```python
from build123d import *

# Parameters (mm, degrees)
F0_W      = 304.8
F0_H      = 41.91
F1_DEPTH  = 72.39
F3_DEPTH  = 44.45
F4_R      = 9.525
F5_DEPTH  = 52.07
F7_DEPTH  = 42.164
F9_DEPTH  = 43.18
F10_R     = 5.08
F11_R     = 5.08
F12_R     = 1.8364316327
F13_DEPTH = 50.8
F14_R     = 2.0092193571
F15_DEPTH = 50.8


with BuildPart() as f1:
    # F0 (on Top) → F1 (new body)
    with BuildSketch(Plane.XY):
        with Locations((152.4, 20.955)):
            Rectangle(F0_W, F0_H)
    extrude(amount=F1_DEPTH)

    # F2 (on face) → F3 (cut)
    with BuildSketch(Plane.XZ):
        Polygon((304.8, 72.39), (0, 72.39), (304.8, 19.05), align=None)
    extrude(amount=-F3_DEPTH, mode=Mode.SUBTRACT)

    # F4 (on face) → F5 (cut)
    with BuildSketch(Plane(origin=(0, 0, 0), x_dir=(0, -1, 0), z_dir=(-1, 0, 0))):
        with Locations((-20.955, 31.115)):
            Circle(F4_R)
    extrude(amount=-F5_DEPTH, mode=Mode.SUBTRACT)

    # F6 (on face) → F7 (cut)
    with BuildSketch(Plane.XZ):
        Polygon((0, 72.39), (0, 53.7492334843), (68.9350515604, 53.7492334843), (95.2856466174, 29.7941416502), (207.8745663166, 29.7941416502), (304.8, 0), (304.8, 19.05), align=None)
    extrude(amount=-F7_DEPTH, mode=Mode.SUBTRACT)

    # F8 (on face) → F9 (cut)
    with BuildSketch(Plane.XZ):
        Polygon((0, 53.7492334843), (0, 46.6843768954), (65.1628002524, 46.6843768954), (95.2856466174, 21.5315297246), (207.8745663166, 21.5315297246), (304.8, 0), (207.8745663166, 29.7941416502), (95.2856466174, 29.7941416502), (68.9350515604, 53.7492334843), align=None)
    extrude(amount=-F9_DEPTH, mode=Mode.SUBTRACT)

    # F10
    f10_edges = [f1.edges().sort_by_distance(p)[0] for p in [
        (152.4, 0, 0),
        (256.337283, 0, 10.765765),
        (151.580106, 0, 21.53153),
        (80.224223, 0, 34.107953),
        (32.5814, 0, 46.684377),
        (0, 0, 23.342188),
    ]]
    fillet(f10_edges, radius=F10_R)

    # F11
    f11_edges = [f1.edges().sort_by_distance(p)[0] for p in [
        (152.4, 41.91, 0),
        (0, 41.91, 23.342188),
        (32.5814, 41.91, 46.684377),
        (80.224223, 41.91, 34.107953),
        (151.580106, 41.91, 21.53153),
        (256.337283, 41.91, 10.765765),
    ]]
    fillet(f11_edges, radius=F11_R)

    # F12 (on face) → F13 (cut)
    with BuildSketch(Plane.XZ):
        with Locations((63.3207473448, 9.5940940082)):
            Circle(F12_R)
    extrude(amount=-F13_DEPTH, mode=Mode.SUBTRACT)

    # F14 (on face) → F15 (cut)
    with BuildSketch(Plane.XZ):
        with Locations((207.3171118243, 8.7452335283)):
            Circle(F14_R)
    extrude(amount=-F15_DEPTH, mode=Mode.SUBTRACT)


solid = f1.part
```
CAD build for the part. Positions are in the model's coordinates, mm. A direction names the side the tool comes from. Round coordinates to 2 decimals unless told otherwise and drop trailing zeros. Order: outer loops, then holes, each group sorted by start corner. A loop starts at its lowest first (then second) coordinate and runs counter-clockwise, first axis right, second up.
Item 1: Saw through at D-D on y = 8. Write the cut outline in (x, z).
Item 2: Saw through at B-B on y = 19.5. Write the cut outline in (x, z).
Item 3: Pin check, flat tips, straight feed: pin 1 (5 mm diameter, centred on x = 207.32, z = 8.75, fed in from +Y); pin 2 (16 mm diameter, centred on x = 154.5, y = 22, fed in from +Z); pin 3 (6 mm diameter, centred on y = 19.5, z = 33, fed in from -X). Stop position of each tip, or through.
Item 4: Saw through at A-A on x = 26.5. Write the cut outline in (y, z) (3 decimals), then the cut area to 3 significant figures.
Item 5: Tool access for faces 1 (the face through (52.07, 21, 31)), 2 (the face through (32, 21, 46.684)), 3 (the face through (151.46, 1.449, 20.004)): list every direction of +Z, -Z, +X, -X, +Y, -Y with a clear straight run to the whole face (end or side of a thin tool).
Item 6: Probe line 1 along Y through (x, z) = (42, 31); line 2 along Z through (x, y) = (159.5, 8); line 3 along Z through (x, y) = (206, 17). List the from-to ranges inside material, lowest first.
Item 7: Saw through at C-C on x = 192.5. Write the cut outline in (y, z).
Reported:
1. outline: (0, 0) - (304.8, 0) - (207.87, 21.53) - (95.29, 21.53) - (65.16, 46.68) - (0, 46.68) - close; hole circle Ø3.67 at (63.32, 9.59); hole circle Ø4.02 at (207.32, 8.75)
2. outline: (0, 0) - (304.8, 0) - (207.87, 21.53) - (95.29, 21.53) - (65.16, 46.68) - (0, 46.68) - (0, 40.53) - (52.07, 40.53) - (52.07, 21.7) - (0, 21.7) - close; hole circle Ø3.67 at (63.32, 9.59); hole circle Ø4.02 at (207.32, 8.75)
3. pin 1: stops at y = 41.91
3. pin 2: stops at z = 21.53
3. pin 3: stops at x = 52.07
4. outline: (0, 5.08) arc R5.08 ccw to (5.08, 0) - (36.83, 0) arc R5.08 ccw to (41.91, 5.08) - (41.91, 41.604) arc R5.08 ccw to (36.83, 46.684) - (5.08, 46.684) arc R5.08 ccw to (0, 41.604) - close; hole circle Ø19.05 at (20.955, 31.115)
4. area: 1,650 mm2
5. face 1: -X
5. face 2: +Z, +X, -X, +Y, -Y
5. face 3: +Z, +X, -Y
6. line 1: y = 0 to 11.43, 30.48 to 41.91
6. line 2: z = 0 to 21.53
6. line 3: z = 0 to 7.23, 10.26 to 21.53
7. outline: (0, 5.08) arc R5.08 ccw to (5.08, 0) - (36.83, 0) arc R5.08 ccw to (41.91, 5.08) - (41.91, 16.45) arc R5.08 ccw to (36.83, 21.53) - (5.08, 21.53) arc R5.08 ccw to (0, 16.45) - close
